Source: CAD feature listing. Evaluate the final solid. Frame: model axes, mm. A direction names the side the tool comes from. Give positions to 0.01 mm unless a question says otherwise; leave off trailing zeros. Order: outer loops, then holes, each group sorted by start corner. A loop starts at its lowest first (then second) coordinate and runs counter-clockwise, first axis right, second up. Notation, with made-up numbers: M 74,40 L 129,40 A24 ccw 129,67 Z; hole C 21.5,53.25 d3. An arc over 180 degrees is marked long. Return JSON: item names as keys, results as strings.
Autodesk Inventor part; units mm, degrees
ref_plane "YZ Plane" through (0, 0, 0) normal (1, 0, 0) x (0, 1, 0)
ref_plane "XZ Plane" through (0, 0, 0) normal (0, 1, 0) x (-1, 0, 0)
ref_plane "XY Plane" through (0, 0, 0) normal (0, 0, 1) x (1, 0, 0)
sketch "Sketch1" plane through (0, 0, 0) normal (0, 1, 0) x (-1, 0, 0)
  circle A0 centre (0, 0) radius 41
  circle A1 centre (0, 0) radius 39
  dimension "d0" = 82
  dimension "d1" = 78
extrude "Extrusion1" add sketch "Sketch1" along normal blind 65
sketch "Sketch2" plane through (0, 65, 0) normal (0, 1, 0) x (1, 0, 0)
  line L0 (-4, -41) -> (4, -41)
  line L1 (4, -41) -> (4, 41)
  line L2 (4, 41) -> (-4, 41)
  line L3 (-4, 41) -> (-4, -41)
  line L4 (-4, -41) -> (4, 41) construction
  line L5 (4, -41) -> (-4, 41) construction
  point P0 (0, 0)
  dimension "d4" = 8
  dimension "d5" = 82
extrude "Extrusion2" cut sketch "Sketch2" against normal blind 5
sketch "Sketch3" plane through (0, 65, 0) normal (0, 1, 0) x (1, 0, 0)
  line L0 (-41, 3) -> (-41, -3)
  line L1 (-41, -3) -> (41, -3)
  line L2 (41, -3) -> (41, 3)
  line L3 (41, 3) -> (-41, 3)
  line L4 (-41, 3) -> (41, -3) construction
  line L5 (-41, -3) -> (41, 3) construction
  line L6 (-41, 3) -> (-35, 3) construction
  point P0 (0, 0)
  dimension "d8" = 6
  dimension "d9" = 90
  dimension "d10" = 82
extrude "Extrusion3" cut sketch "Sketch3" against normal blind 5
sketch "Sketch4" plane through (0, 65, 0) normal (0, 1, 0) x (1, 0, 0)
  line L0 (0, 0) -> (0, 13)
  line L1 (0, 13) -> (0, -13)
  line L2 (0, -13) -> (82, -13)
  line L3 (82, -13) -> (82, 13)
  line L4 (82, 13) -> (0, 13)
  dimension "d13" = 13
  dimension "d14" = 26
  dimension "d15" = 82
extrude "Extrusion4" cut sketch "Sketch4" against normal blind 30
sketch "Sketch5" plane through (0, 0, 0) normal (1, 0, 0) x (0, 1, 0)
  circle A0 centre (0, 0) radius 4
  dimension "d18" = 8
extrude "Extrusion5" cut sketch "Sketch5" against normal blind 82
properties part number "case"
1. Section query A-A (x = 0). Return loops of the section in (y, z).
Evaluation:
{"outline": "M 0,-41 L 60,-41 L 60,-39 L 0,-39 Z; M 0,39 L 60,39 L 60,41 L 0,41 Z"}
2. Section query C-C (y = 8). Return loops of the section in (x, z).
Evaluation:
{"outline": "C 0,0 d82; hole C 0,0 d78"}
3. Ray query, probe 1 along Z at (x, y) = (-4, 10); probe 2 along Z at (x, y) = (0, 28). Return the intervals inside material, ascending.
Evaluation:
{"probe 1": "z = -40.8 to -38.79, 38.79 to 40.8", "probe 2": "z = -41 to -39, 39 to 41"}
4. First-contact query: pin 1 (12 mm diameter, centred on x = -12, y = 11, fed in from +Z); pin 2 (6 mm diameter, centred on x = 15, y = 37.5, fed in from -Z); pin 3 (1.8 mm diameter, centred on x = 2, z = 40, fed in from +Y); pin 4 (10 mm diameter, centred on x = -28, z = 19, fed in from +Y). Flat tips, straight axial feed; report the tip coordinate or a pass-through.
Evaluation:
{"pin 1": "stops at z = 40.56", "pin 2": "stops at z = -39.2", "pin 3": "stops at y = 60", "pin 4": "passes through"}
5. Set-up query: faces 1 (the face through (4, 63, 40)), 2 (the face through (-40, 60, 0)), 3 (the face through (38, 50, 13)). Return all of +Z, -Z, +X, -X, +Y, -Y with unobstructed straight access to the full face (end or side cutting, diameter ignored); none if empty.
Evaluation:
{"face 1": "+Z, -Z, +Y", "face 2": "+X, -X, +Y", "face 3": "+X, +Y"}
6. Draft query along X for faces 4 (the face through (25.4, 65, -29.9)), 5 (the face through (-37.874, 32.045, 15.703)), 6 (the face through (-4, 63, -40)). Return one class per face: pulls with the +X half, pulls with the -X half, needs draft (parallel to the pull), parting line crosses it, or undercut.
Evaluation:
{"face 4": "needs draft", "face 5": "parting line crosses it", "face 6": "undercut"}
7. Section query D-D (y = 43). Return loops of the section in (x, z), then the cut area to 3 significant figures.
Evaluation:
{"outline": "M 36.77,-13 A39 cw long 36.77,13 L 38.88,13 A41 ccw long 38.88,-13 Z", "area": "450 mm^2"}
8. Section query B-B (z = 0). Return loops of the section in (x, y).
Evaluation:
{"outline": "M -41,4 L -39,4 L -39,60 L -41,60 Z; M 39,0 L 41,0 L 41,35 L 39,35 Z"}
